Answer from the drawing. Dimensions are ordinates in mm from the lowest x, y and z of the part. A direction names the side the tool comes from. Give positions to 0.01 mm unless a question says otherwise; leave off trailing zeros. Order: outer loops, then holes, each group sorted by start corner. A loop starts at its lowest first (then second) coordinate and runs counter-clockwise, first axis right, second up. Notation, with made-up numbers: (79.25, 65.25) - (100.25, 65.25) arc R7 cw to (100.25, 71.25) - close; hole circle Ø4 at (19.25, 22.25). An arc over 180 degrees is marked (long way). Write each question's results on one line, items separated by ' | '.
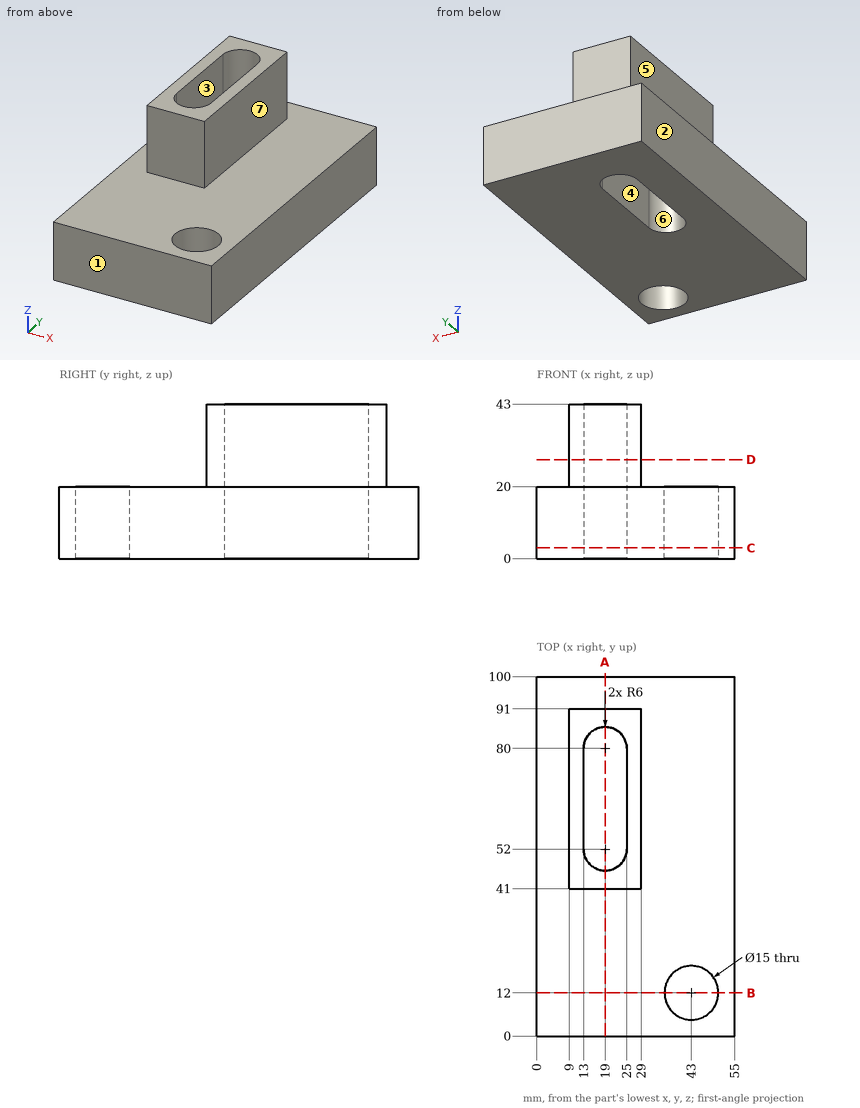
(1) The mould has two halves that part along X. Classify the marked faces 1, 2, 3 and 4: pulls with the +X half, pulls with the -X half, needs draft (parallel to the pull), parting line crosses it, or undercut.
Conclusion:
face 1: needs draft | face 2: pulls with the -X half | face 3: undercut | face 4: undercut
(2) For the marked faces 5, 6 and 7, determine the directions among +Z, -Z, +X, -X, +Y, -Y from which every point of the face is accessible in a straight line to the end or side of a thin tool.
Conclusion:
face 5: +Z, -X, +Y, -Y | face 6: +Z, -Z | face 7: +Z, +X, +Y, -Y
(3) Section C-C (z = 3) is taken. Give the vertices of the cut face in (x, y), plus the area to 3 significant figures.
Conclusion:
outline: (0, 0) - (55, 0) - (55, 100) - (0, 100) - close; hole (13, 52) arc R6 ccw to (25, 52) - (25, 80) arc R6 ccw to (13, 80) - close; hole circle Ø15 at (43, 12) | area: 4,870 mm^2
(4) Section A-A (x = 19) is taken. Give the vertices of the cut face in (y, z), plus the area to 3 significant figures.
Conclusion:
outline: (0, 0) - (46, 0) - (46, 43) - (41, 43) - (41, 20) - (0, 20) - close; (86, 0) - (100, 0) - (100, 20) - (91, 20) - (91, 43) - (86, 43) - close | area: 1,430 mm^2
(5) Section B-B (y = 12) is taken. Give the vertices of the cut face in (x, z), plus the area to 3 significant figures.
Conclusion:
outline: (0, 0) - (35.5, 0) - (35.5, 20) - (0, 20) - close; (50.5, 0) - (55, 0) - (55, 20) - (50.5, 20) - close | area: 800 mm^2
(6) Consider probe 1 along X at (y, z) = (51.5, 6); probe 2 along Y at (x, z) = (43, 7.75); probe 3 along X at (y, z) = (74.5, 28.5). Determine where each line is inside the solid, lowest interval first. Write a range as [from, to].
Conclusion:
probe 1: [0, 13.02], [24.98, 55] | probe 2: [0, 4.5], [19.5, 100] | probe 3: [9, 13], [25, 29]
(7) Each of these flat-tipped pins is pushed along its axis until it touches: pin 1 (3 mm diameter, centred on x = 47.5, y = 75.5, fed in from +Z); pin 2 (11.5 mm diameter, centred on y = 60.5, z = 37, fed in from +X); pin 3 (3 mm diameter, centred on x = 25.5, z = 36, fed in from -Y). Where does it stop, or does it pass through?
Conclusion:
pin 1: z = 20 | pin 2: x = 29 | pin 3: y = 41
(8) Section D-D (z = 27.5) is taken. Give the vertices of the cut face in (x, y), plus the area to 3 significant figures.
Conclusion:
outline: (9, 41) - (29, 41) - (29, 91) - (9, 91) - close; hole (13, 52) arc R6 ccw to (25, 52) - (25, 80) arc R6 ccw to (13, 80) - close | area: 551 mm^2
